Verification items for the finished model (mm, model axes). A direction names the side the tool comes from. Coordinates: 2 decimals unless noted, no trailing zeros. Loops run counter-clockwise (first coordinate to the right, second up) from the corner with the lowest first, then second, coordinate; pieces in that order, holes last. Notation, with made-up numbers: (-11.75, -18.75) -> (24.25, -18.75) arc R13 cw to (24.25, 4.25) -> close; hole circle Ø7 at (87.25, 54). An arc over 180 degrees is marked (long way). Write item = value, one per line.
```python
from build123d import *

# Parameters (mm, degrees)
BOSS_EXTRUDE1_DEPTH = 20
SKETCH14_W          = 65.5
SKETCH14_H          = 14
BOSS_EXTRUDE2_DEPTH = 20
SKETCH13_R          = 1.5
CUT_EXTRUDE2_DEPTH  = 54
SKETCH12_R          = 5
CUT_EXTRUDE3_DEPTH  = 4


with BuildPart() as part:
    # Sketch1 → Boss-Extrude1 (new body)
    with BuildSketch(Plane.XY):
        Polygon((26.75, 14), (26.75, 6), (38.75, 6), (38.75, 14), (65.5, 14), (65.5, 0), (0, 0), (0, 14), align=None)
    extrude(amount=BOSS_EXTRUDE1_DEPTH)

    # Sketch14 → Boss-Extrude2 (add)
    with BuildSketch(Plane.XY):
        with Locations((32.75, 7)):
            Rectangle(SKETCH14_W, SKETCH14_H)
    extrude(amount=BOSS_EXTRUDE2_DEPTH)

    # Sketch13 → Cut-Extrude2 (cut)
    with BuildSketch(Plane.XZ):
        with Locations(Location((5.05, 7.05, 0), (0, 0, 270))):
            Circle(SKETCH13_R)
        with Locations(Location((5.05, 13.55, 0), (0, 0, 270))):
            Circle(SKETCH13_R)
        with Locations(Location((60.45, 7.05, 0), (0, 0, 270))):
            Circle(SKETCH13_R)
        with Locations(Location((60.45, 13.55, 0), (0, 0, 270))):
            Circle(SKETCH13_R)
    extrude(amount=-CUT_EXTRUDE2_DEPTH, mode=Mode.SUBTRACT)

    # Sketch12 → Cut-Extrude3 (cut)
    with BuildSketch(Plane(origin=(0, 14, 0), x_dir=(1, 0, 0), z_dir=(0, 1, 0))):
        with Locations(Location((17.75, -10, 0), (0, 0, 270))):
            Circle(SKETCH12_R)
        with Locations(Location((47.75, -10, 0), (0, 0, 90))):
            Circle(SKETCH12_R)
    extrude(amount=-CUT_EXTRUDE3_DEPTH, mode=Mode.SUBTRACT)


solid = part.part
```
1) Sectioned sample at C-C, the plane z = 13.75. Record the cut outline in (x, y), plus the area to 3 significant figures.
Ans:
outline = (0, 0) -> (3.56, 0) -> (3.56, 14) -> (0, 14) -> close; (6.54, 0) -> (58.96, 0) -> (58.96, 14) -> (51.06, 14) -> (51.06, 10) -> (44.44, 10) -> (44.44, 14) -> (21.06, 14) -> (21.06, 10) -> (14.44, 10) -> (14.44, 14) -> (6.54, 14) -> close; (61.94, 0) -> (65.5, 0) -> (65.5, 14) -> (61.94, 14) -> close
area = 781 mm2
2) Sectioned sample at D-D, the plane x = 47.75. Record the cut outline in (y, z).
Ans:
outline = (0, 0) -> (14, 0) -> (14, 5) -> (10, 5) -> (10, 15) -> (14, 15) -> (14, 20) -> (0, 20) -> close
3) Depth check by flat-ended pin: pin 1 Ø4 at (x, z) = (5.05, 7.05) entering from -Y; pin 2 Ø5 at (x, z) = (48, 10) entering from +Y. Enter the tip coordinate at first touch or a pass-through.
Ans:
pin_1 = 0
pin_2 = 10
4) Sectioned sample at B-B, the plane y = 9. Record the cut outline in (x, z).
Ans:
outline = (0, 0) -> (65.5, 0) -> (65.5, 20) -> (0, 20) -> close; hole circle Ø3 at (5.05, 7.05); hole circle Ø3 at (5.05, 13.55); hole circle Ø3 at (60.45, 7.05); hole circle Ø3 at (60.45, 13.55)
5) Sectioned sample at A-A, the plane x = 60.45. Record the cut outline in (y, z), plus the area to 3 significant figures.
Ans:
outline = (0, 0) -> (14, 0) -> (14, 5.55) -> (0, 5.55) -> close; (0, 8.55) -> (14, 8.55) -> (14, 12.05) -> (0, 12.05) -> close; (0, 15.05) -> (14, 15.05) -> (14, 20) -> (0, 20) -> close
area = 196 mm2
6) Material ranges on line 1 (X direction, y = 7.25, z = 7.05); line 2 (X direction, y = 11, z = 7.05); line 3 (X direction, y = 7.25, z = 14.5), recorded low to high.
Ans:
line_1 = 0 to 3.55, 6.55 to 58.95, 61.95 to 65.5
line_2 = 0 to 3.55, 6.55 to 13.71, 21.79 to 43.71, 51.79 to 58.95, 61.95 to 65.5
line_3 = 0 to 3.89, 6.21 to 59.29, 61.61 to 65.5
7) Release check for a two-part mould opening along Z. For faces 3 (the face through (0, 7, 10)), 4 (the face through (33, 7, 0)), 5 (the face through (33, 7, 20)), 6 (the face through (18, 10, 10)) record: pulls with the +Z half, pulls with the -Z half, needs draft (parallel to the pull), parting line crosses it, or undercut.
Ans:
face_3 = needs draft
face_4 = pulls with the -Z half
face_5 = pulls with the +Z half
face_6 = undercut
8) Tool access check on faces 1 (the face through (13.314, 12.028, 12.307)), 2 (the face through (61.937, 6.902, 13.745)). Record the directions out of +Z, -Z, +X, -X, +Y, -Y that give a thin tool (end or side, any length) a straight path to the whole face; none if there is none.
Ans:
face_1 = +Y
face_2 = +Y, -Y
